Autodesk Inventor part; units mm, degrees
ref_plane "YZ Plane" through (0, 0, 0) normal (1, 0, 0) x (0, 1, 0)
ref_plane "XZ Plane" through (0, 0, 0) normal (0, 1, 0) x (-1, 0, 0)
ref_plane "XY Plane" through (0, 0, 0) normal (0, 0, 1) x (1, 0, 0)
sketch "Sketch1" plane through (0, 0, 0) normal (0, 1, 0) x (-1, 0, 0)
  circle A0 centre (0, 0) radius 38.1 construction
  line L0 (0, 0) -> (38.1, 0) construction
  line L1 (0, 0) -> (-38.1, 0) construction
  circle A1 centre (38.1, 0) radius 1.905
  circle A2 centre (-38.1, 0) radius 1.905
  circle A3 centre (38.1, 0) radius 9.525
  circle A4 centre (-38.1, 0) radius 9.525
  line L2 (0, 0) -> (0, 44.45) construction
  circle A5 centre (0, 44.45) radius 76.2 construction
  circle A6 centre (0, 44.45) radius 19.05 construction
  circle A7 centre (0, 0) radius 25.4 construction
  circle A8 centre (0, 44.45) radius 4.7625
  circle A9 centre (0, 44.45) radius 22.225
  line L3 (19.6103, 54.9088) -> (46.5044, 4.4824)
  line L4 (-19.6103, 54.9088) -> (-46.5044, 4.4824)
  line L5 (13.153, 26.535) -> (29.6956, -4.4824)
  line L6 (-13.153, 26.535) -> (-29.6956, -4.4824)
  circle A10 centre (0, 44.45) radius 15.875 construction
  circle A11 centre (0, 60.325) radius 1.905
  circle A12 centre (-13.7482, 52.3875) radius 1.905
  circle A13 centre (-13.7482, 36.5125) radius 1.905
  circle A14 centre (0, 28.575) radius 1.905
  circle A15 centre (13.7482, 36.5125) radius 1.905
  circle A16 centre (13.7482, 52.3875) radius 1.905
  circle A17 centre (0, -19.05) radius 4.7625
  circle A18 centre (0, -19.05) radius 8 construction
  circle A19 centre (0, -19.05) radius 9.5 construction
  line L7 (0, -19.05) -> (9.5, -19.05) construction
  line L8 (0, -19.05) -> (6.7175, -12.3325) construction
  circle A20 centre (5.6569, -13.3931) radius 1.5
  line L9 (0, -19.05) -> (6.7175, -25.7675) construction
  circle A21 centre (6.7175, -25.7675) radius 1.5
  circle A22 centre (-6.7175, -12.3325) radius 1.5
  circle A23 centre (-5.6569, -24.7069) radius 1.5
  circle A24 centre (0, -19.05) radius 15.875
  line L10 (9.1369, -32.032) -> (43.5821, -7.7892)
  line L11 (14.5471, -12.6942) -> (28.7456, -2.7012)
  line L12 (-9.1369, -32.032) -> (-43.5821, -7.7892)
  line L13 (-14.5471, -12.6942) -> (-28.7456, -2.7012)
  point P0 (-29.6956, -4.4824)
  point P1 (29.6956, -4.4824)
  dimension "d14" = 31.75
  dimension "d22" = 16
  dimension "d0" = 76.2
  dimension "d1" = 3.81
  dimension "d2" = 3.81
  dimension "d3" = 19.05
  dimension "d4" = 19.05
  dimension "d5" = 152.4
  dimension "d6" = 38.1
  dimension "d7" = 50.8
  dimension "d8" = 9.525
  dimension "d9" = 44.45
  dimension "d10" = 19.05
  dimension "d15" = 3.81
  dimension "d18" = 360
  dimension "d20" = 9.525
  dimension "d21" = 63.5
  dimension "d23" = 19
  dimension "d24" = 45
  dimension "d25" = 3
  dimension "d26" = 3
  dimension "d29" = 360
  dimension "d31" = 31.75
  dimension "d32" = 12.7
extrude "Extrusion1" add sketch "Sketch1" along normal blind 4.7625 contours A3 | A3 L5 A9 L3 | L10 A24 L11 L5 A3 | A9 | A24 | A9 L6 A4 L4 | L12 A4 L6 L13 A24 | A4
fillet "Fillet1" radius 6.35 6 edges at (-13.153, 2.3813, 26.535) (13.153, 2.3813, 26.535) (-14.5471, 2.3813, -12.6942) (-28.7456, 2.3813, -2.7012) (14.5471, 2.3813, -12.6942) (28.7456, 2.3813, -2.7012)
equation "\"d2\" = d1"
equation "\"d4\" = d3"
properties part number "Upright - Bottom" material "Aluminum 6061"
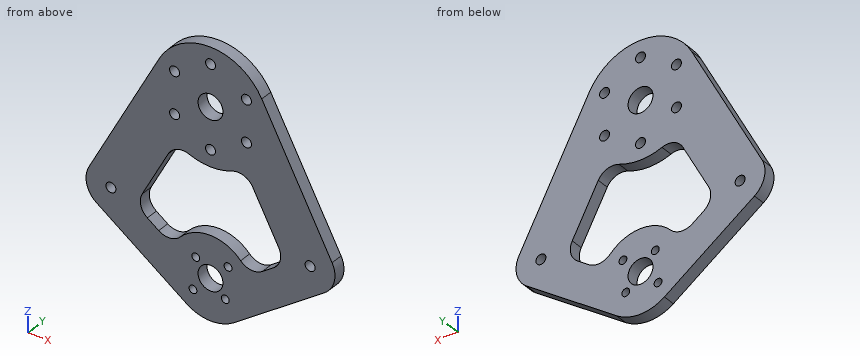
Input: part model. Units: mm. Frame: model coordinates. Give positions to 0.01 mm unless a question says otherwise; leave off trailing zeros. Order: outer loops, then holes, each group sorted by start corner. A loop starts at its lowest first (then second) coordinate and runs counter-clockwise, first axis right, second up. Notation, with made-up numbers: M 29.5,-35.75 L 88.5,-35.75 A15 ccw 88.5,-13.75 Z; hole C 79.25,77 d7. An arc over 180 degrees is marked long. Return JSON: item names as keys, results as strings.
Item 1: Cut plane B-B (z = 0). Return loops of the section in (x, y) (1 decimal), then the cut area to 3 significant figures.
Solutions:
{"outline": "M -47.6,0 L -40,0 L -40,4.8 L -47.6,4.8 Z; M -36.2,0 L -26.8,0 L -26.8,4.8 L -36.2,4.8 Z; M 26.8,0 L 36.2,0 L 36.2,4.8 L 26.8,4.8 Z; M 40,0 L 47.6,0 L 47.6,4.8 L 40,4.8 Z", "area": "162 mm^2"}
Item 2: Cut plane D-D (z = 14). Return loops of the section in (x, y), then the cut area to 3 significant figures.
Solutions:
{"outline": "M -41.43,0 L -19.84,0 L -19.84,4.76 L -41.43,4.76 Z; M 19.84,0 L 41.43,0 L 41.43,4.76 L 19.84,4.76 Z", "area": "206 mm^2"}
Item 3: First-contact query: P1, Ø5, axis at x = 23.5, z = 0, coming from the +Y side. Flat tip, straight axial feed; report the tip coordinate or a pass-through.
Solutions:
{"P1": "through"}
Item 4: Cut plane C-C (x = 22). Return loops of the section in (y, z), then the cut area to 3 significant figures.
Solutions:
{"outline": "M 0,-22.98 L 4.76,-22.98 L 4.76,-7.45 L 0,-7.45 Z; M 0,9.95 L 4.76,9.95 L 4.76,50.43 L 0,50.43 Z", "area": "267 mm^2"}
Item 5: Ray query, probe 1 along Z at (x, y) = (13.5, 3.75); probe 2 along X at (y, z) = (3.55, -13); probe 3 along X at (y, z) = (0.3, 61). Return the intervals inside material, ascending.
Solutions:
{"probe 1": "-28.96 to -9.56, 23.53 to 34.62, 38.4 to 50.5, 54.28 to 62.11", "probe 2": "-36.18 to -7.1, -4.21 to 5.37, 8.06 to 36.18", "probe 3": "-14.83 to -1.78, 1.78 to 14.83"}
Item 6: Cut plane A-A (x = 0). Return loops of the section in (y, z) (1 decimal), then the cut area to 3 significant figures.
Solutions:
{"outline": "M 0,-34.9 L 4.8,-34.9 L 4.8,-23.8 L 0,-23.8 Z; M 0,-14.3 L 4.8,-14.3 L 4.8,-3.2 L 0,-3.2 Z; M 0,22.2 L 4.8,22.2 L 4.8,26.7 L 0,26.7 Z; M 0,30.5 L 4.8,30.5 L 4.8,39.7 L 0,39.7 Z; M 0,49.2 L 4.8,49.2 L 4.8,58.4 L 0,58.4 Z; M 0,62.2 L 4.8,62.2 L 4.8,66.7 L 0,66.7 Z", "area": "236 mm^2"}
